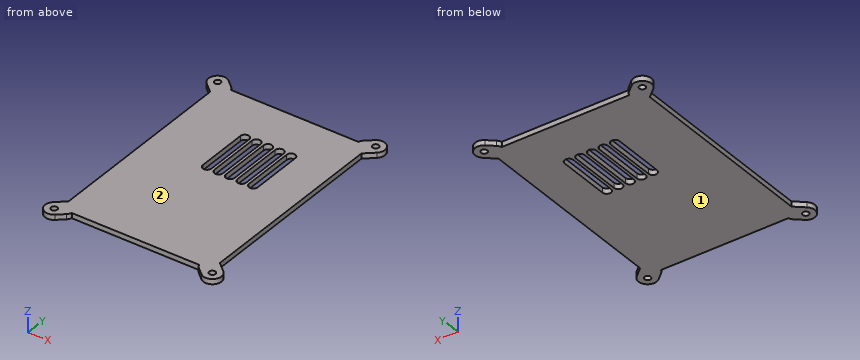
Autodesk Inventor part; units mm, degrees
ref_plane "YZ Plane" through (0, 0, 0) normal (1, 0, 0) x (0, 1, 0)
ref_plane "XZ Plane" through (0, 0, 0) normal (0, 1, 0) x (-1, 0, 0)
ref_plane "XY Plane" through (0, 0, 0) normal (0, 0, 1) x (1, 0, 0)
ref_plane "Work Plane1" through (0, 0, 0) normal (0, 0, 1) x (1, 0, 0)
sketch "Sketch1" plane through (0, 0, 0) normal (0, 0, 1) x (1, 0, 0)
  line L0 (162.668, -44.5954) -> (162.668, 41.2818)
  line L1 (166.8059, 44.8966) -> (162.668, 41.2818)
  arc A0 (166.8059, 44.8966) -> (161.5426, 50.9214) centre (164.1742, 47.909) ccw
  circle A1 centre (164.1742, 47.909) radius 1.375
  line L2 (158.5302, 48.2898) -> (161.5426, 50.9214)
  arc A2 (158.5302, 48.2898) -> (157.3844, 46.5932) centre (161.1618, 45.2774) ccw
  line L3 (157.3844, 46.5932) -> (101.3516, 46.5932)
  arc A3 (101.3516, 46.5932) -> (100.2059, 48.2898) centre (97.5742, 45.2774) ccw
  line L4 (97.1935, 50.9214) -> (100.2059, 48.2898)
  arc A4 (97.1935, 50.9214) -> (91.9302, 44.8966) centre (94.5618, 47.909) ccw
  circle A5 centre (94.5618, 47.909) radius 1.375
  line L5 (96.068, 41.2818) -> (91.9302, 44.8966)
  line L6 (96.068, 41.2818) -> (96.068, -44.5954)
  line L7 (91.9302, -48.2102) -> (96.068, -44.5954)
  arc A6 (91.9302, -48.2102) -> (97.1935, -54.235) centre (94.5618, -51.2226) ccw
  line L8 (100.2059, -51.6034) -> (97.1935, -54.235)
  arc A7 (100.2059, -51.6034) -> (101.3516, -49.9068) centre (97.5742, -48.591) ccw
  circle A8 centre (94.5618, -51.2226) radius 1.375
  line L9 (101.3516, -49.9068) -> (157.3844, -49.9068)
  line L10 (161.5426, -54.235) -> (158.5302, -51.6034)
  arc A9 (157.3844, -49.9068) -> (158.5302, -51.6034) centre (161.1618, -48.591) ccw
  arc A10 (161.5426, -54.235) -> (166.8059, -48.2102) centre (164.1742, -51.2226) ccw
  line L11 (162.668, -44.5954) -> (166.8059, -48.2102)
  circle A11 centre (164.1742, -51.2226) radius 1.375
  line L12 (102.868, 42.7932) -> (155.868, 42.7932)
  arc A12 (158.868, 39.7932) -> (155.868, 42.7932) centre (155.868, 39.7932) ccw
  line L13 (158.868, 39.7932) -> (158.868, -43.1068)
  arc A13 (155.868, -46.1068) -> (158.868, -43.1068) centre (155.868, -43.1068) ccw
  line L14 (155.868, -46.1068) -> (102.868, -46.1068)
  arc A14 (99.868, -43.1068) -> (102.868, -46.1068) centre (102.868, -43.1068) ccw
  line L15 (99.868, -43.1068) -> (99.868, 39.7932)
  arc A15 (102.868, 42.7932) -> (99.868, 39.7932) centre (102.868, 39.7932) ccw
  point P0 (0, 0)
  point P1 (-32.2078, 42.9557)
  point P2 (-31.0209, 50.8588)
  point P3 (-31.2556, 42.9706)
  point P4 (90.7091, 46.8336)
  point P5 (90.8754, -49.6701)
  point P6 (94.8543, -45.6557)
  point P7 (38.6589, -48.4904)
  point P8 (35.6268, 48.0781)
extrude "Extrusion1" add sketch "Sketch1" along normal blind 2.25 contours L11 A10 L10 A9 L9 A7 L8 A6 L7 L6 L5 A4 L4 A3 L3 A2 L2 A0 L1 L0 | A1 | A5 | A8 | A11 | L12 A12 L13 A13 L14 A14 L15 A15
sketch "Sketch2" plane through (0, 0, 2.25) normal (0, 0, 1) x (1, 0, 0)
  line L0 (140.3574, 20.4135) -> (126.2672, 20.4135) construction
  line L1 (126.2672, 20.4135) -> (126.2672, 6.3233) construction
  line L2 (126.2672, 6.3233) -> (140.3574, 6.3233) construction
  line L3 (140.3574, 6.3233) -> (140.3574, 20.4135) construction
  line L4 (133.3123, 25.0032) -> (133.3123, 2.1432) construction
  line L5 (131.4073, 25.0032) -> (131.4073, 2.1432)
  line L6 (135.2173, 2.1432) -> (135.2173, 25.0032)
  arc A0 (135.2173, 25.0032) -> (131.4073, 25.0032) centre (133.3123, 25.0032) ccw
  arc A1 (131.4073, 2.1432) -> (135.2173, 2.1432) centre (133.3123, 2.1432) ccw
  line L7 (162.668, -44.5954) -> (162.668, 41.2818)
  line L8 (157.3844, 46.5932) -> (101.3516, 46.5932)
  line L9 (140.2973, 2.1432) -> (140.2973, 25.0032)
  arc A2 (140.2973, 25.0032) -> (136.4873, 25.0032) centre (138.3923, 25.0032) ccw
  line L10 (136.4873, 25.0032) -> (136.4873, 2.1432)
  arc A3 (136.4873, 2.1432) -> (140.2973, 2.1432) centre (138.3923, 2.1432) ccw
  line L11 (145.3773, 2.1432) -> (145.3773, 25.0032)
  arc A4 (145.3773, 25.0032) -> (141.5673, 25.0032) centre (143.4723, 25.0032) ccw
  line L12 (141.5673, 25.0032) -> (141.5673, 2.1432)
  arc A5 (141.5673, 2.1432) -> (145.3773, 2.1432) centre (143.4723, 2.1432) ccw
  arc A6 (130.1373, 25.0032) -> (126.3273, 25.0032) centre (128.2323, 25.0032) ccw
  line L13 (130.1373, 2.1432) -> (130.1373, 25.0032)
  line L14 (126.3273, 25.0032) -> (126.3273, 2.1432)
  arc A7 (126.3273, 2.1432) -> (130.1373, 2.1432) centre (128.2323, 2.1432) ccw
  arc A8 (125.0573, 25.0032) -> (121.2473, 25.0032) centre (123.1523, 25.0032) ccw
  line L15 (125.0573, 2.1432) -> (125.0573, 25.0032)
  line L16 (121.2473, 25.0032) -> (121.2473, 2.1432)
  arc A9 (121.2473, 2.1432) -> (125.0573, 2.1432) centre (123.1523, 2.1432) ccw
  circle A10 centre (94.5618, -51.2226) radius 1.375
  circle A11 centre (164.1742, -51.2226) radius 1.375
  circle A12 centre (164.1742, 47.909) radius 1.375
  circle A13 centre (94.5618, 47.909) radius 1.375
  point P0 (0, 0)
  point P1 (133.3123, 13.5732)
  dimension "d2" = 11.43
  dimension "d3" = 3.81
  dimension "d4" = 27.4507
  dimension "d5" = 21.59
  dimension "d6" = 14.0902
  dimension "d7" = 22.3106
  dimension "d8" = 36.4008
  dimension "d9" = 26.1797
  dimension "d12" = 5.08
  dimension "d19" = 5.08
extrude "Extrusion2" cut sketch "Sketch2" against normal up to surface (2.25 mm away)
properties part number "_3DPrint"
Geometry check sheet. Reference: the model listing, model coordinates, mm. Face numbers are marked on the shaded views. Give positions to 0.01 mm unless a question says otherwise; leave off trailing zeros. Order: outer loops, then holes, each group sorted by start corner. A loop starts at its lowest first (then second) coordinate and runs counter-clockwise, first axis right, second up.
1) Draft check along Z on the marked faces 1 and 2. Enter one of: released by +Z, released by -Z, zero draft, split by the parting line, or undercut.
Results are:
face 1: released by -Z
face 2: released by +Z
2) Gauge pin test, flat ends, axial feed: pin 1 (0.7 mm diameter, centred on y = 13, z = 1.5, fed in from +X); pin 2 (1.1 mm diameter, centred on y = -19.5, z = 1.5, fed in from -X). Record the tip position at first contact, or that the pin passes through.
Results are:
pin 1: stops at x = 162.67
pin 2: stops at x = 96.07
3) Cross-section at B-B (z = 1.5). Give the number of separate pieces and of enclosed holes in the cut face, then the cut area to 3 significant figures.
Results are:
separate pieces: 1
enclosed holes: 9
area: 6,140 mm2
4) Cross-section at C-C (y = -5). Record the boundary of the cut face in (x, z), then the cut area to 3 significant figures.
Results are:
outline: (96.07, 0) - (162.67, 0) - (162.67, 2.25) - (96.07, 2.25) - close
area: 150 mm2
5) Cross-section at A-A (y = 11). Record the boundary of the cut face in (x, z), then the cut area to 3 significant figures.
Results are:
outline: (96.07, 0) - (121.25, 0) - (121.25, 2.25) - (96.07, 2.25) - close; (125.06, 0) - (126.33, 0) - (126.33, 2.25) - (125.06, 2.25) - close; (130.14, 0) - (131.41, 0) - (131.41, 2.25) - (130.14, 2.25) - close; (135.22, 0) - (136.49, 0) - (136.49, 2.25) - (135.22, 2.25) - close; (140.3, 0) - (141.57, 0) - (141.57, 2.25) - (140.3, 2.25) - close; (145.38, 0) - (162.67, 0) - (162.67, 2.25) - (145.38, 2.25) - close
area: 107 mm2
6) Material ranges on probe 1 along X at (y, z) = (15, 0.5); probe 2 along Y at (x, z) = (95, 1.5); probe 3 along X at (y, z) = (-51, 0.5), recorded low to high.
Results are:
probe 1: x = 96.07 to 121.25, 125.06 to 126.33, 130.14 to 131.41, 135.22 to 136.49, 140.3 to 141.57, 145.38 to 162.67
probe 2: y = -55.2 to -52.53, -49.92 to -45.53, 42.21 to 46.61, 49.21 to 51.88
probe 3: x = 90.57 to 93.2, 95.92 to 100.77, 157.97 to 162.82, 165.53 to 168.17
